Work out the finished part from the listing and answer in its coordinate system (mm). A direction names the side the tool comes from. Coordinates: 2 decimals unless noted, no trailing zeros. Write each loop counter-clockwise with the first axis right and the second up, starting at its lowest first coordinate (ties: lowest second). Pieces come first, ordered by that corner, then holes. Notation, with made-up numbers: (1, -6) - (41, -6) arc R5 cw to (41, 3) - close; hole circle Ø7 at (-37.75, -24). An arc over 180 degrees is marked (long way). Answer as a JSON object with one key per item and string values. Group by question number.
from build123d import *
from build123d.topology import SkipClean

# Parameters (mm, degrees)
EXTRUDE_1_DEPTH      = 4
EXTRUDE_1_DEPTH_BACK = 4
FILLET_4_R           = 1
EXTRUDE_2_DEPTH      = 5
FILLET_5_R           = 3
SKETCH_5_R           = 0.2
CUT_EXTRUDE_1_DEPTH  = 54.051861419


with BuildPart() as part:
    # Эскиз1 → Бобышка-Вытянуть1 (new, two sides: drawn at the far end of the back side and taken through both)
    with BuildSketch(Plane(origin=(22.5, -18, -41), x_dir=(0, -1, 0), z_dir=(1, 0, 0)).offset(-EXTRUDE_1_DEPTH_BACK)):
        with BuildLine():
            Line((-51, -2.5), (-51, 0.5))
            Line((-51, 0.5), (-61, 0.5))
            Line((-61, 0.5), (-61, -39.5))
            Line((-61, -39.5), (-51, -39.5))
            Line((-51, -39.5), (-51, -36.5))
            Line((-51, -36.5), (-58, -36.5))
            Line((-58, -36.5), (-58, -33.885132318))
            ThreePointArc((-58, -33.885132318), (-54.5, -35), (-51, -33.885132318))
            Line((-51, -33.885132318), (-51, -30.885132318))
            ThreePointArc((-51, -30.885132318), (-54.5, -32.948640645), (-58, -30.885132318))
            Line((-58, -30.885132318), (-58, -8.114867682))
            ThreePointArc((-58, -8.114867682), (-54.5, -6.051359355), (-51, -8.114867682))
            Line((-51, -8.114867682), (-51, -5.114867682))
            ThreePointArc((-51, -5.114867682), (-54.5, -4), (-58, -5.114867682))
            Line((-58, -5.114867682), (-58, -2.5))
            Line((-58, -2.5), (-51, -2.5))
        make_face()
    extrude(amount=EXTRUDE_1_DEPTH + EXTRUDE_1_DEPTH_BACK)

    # Скругление4
    # the kernel refuses this fillet: 1 mm, written as the material it adds along each edge
    with BuildSketch(Plane(origin=(26.5, 40, -38.5), x_dir=(0, 0, 1), z_dir=(-1, 0, 0)), Plane(origin=(18.5, 40, -4.5), x_dir=(0, 0, -1), z_dir=(1, 0, 0))) as fillet_4_piece_1:
        with BuildLine():
            CenterArc((FILLET_4_R, -FILLET_4_R), FILLET_4_R, 90, 90)
            Line((0, -FILLET_4_R), (0, 0))
            Line((0, 0), (FILLET_4_R, 0))
        make_face()
    extrude(amount=8)
    with BuildSketch(Plane(origin=(26.5, 40, -35.885132318), x_dir=(0, 0, -1), z_dir=(-1, 0, 0))) as fillet_4_piece_2:
        with BuildLine():
            CenterArc((1.65681317, 1), FILLET_4_R, 159.234649254, 110.765350746)
            ThreePointArc((0.721772915, 1.354541568), (0.404005567, 0.654294593), (0, 0))
            Line((0, 0), (1.65681317, 0))
        make_face()
    extrude(amount=8)
    with BuildSketch(Plane(origin=(18.5, 40, -32.885132318), x_dir=(0, -0.5188652741265531, -0.8548560272382577), z_dir=(1, 0, 0))) as fillet_4_piece_3:
        with BuildLine():
            CenterArc((0.281062042, -0.999193595), FILLET_4_R, 87.698857305, 33.557309762)
            Line((-0.237803232, -0.144337567), (0, 0))
            ThreePointArc((0, 0), (0.160606881, 0.003225622), (0.321213762, 0))
        make_face()
    extrude(amount=8)
    with BuildSketch(Plane(origin=(18.5, 40, -10.114867682), x_dir=(0, 0, -1), z_dir=(1, 0, 0))) as fillet_4_piece_4:
        with BuildLine():
            CenterArc((0.278179278, -1), FILLET_4_R, 90, 33.557309762)
            ThreePointArc((-0.27459152, -0.166666667), (-0.138969423, -0.080575891), (0, 0))
            Line((0, 0), (0.278179278, 0))
        make_face()
    extrude(amount=8)
    with BuildSketch(Plane(origin=(18.5, 40, -7.114867682), x_dir=(0, -0.8825285241752726, 0.4702588691529541), z_dir=(1, 0, 0))) as fillet_4_piece_5:
        with BuildLine():
            CenterArc((1.661659612, -0.991926012), FILLET_4_R, 97.285750856, 110.765350746)
            Line((0.779131087, -1.462184881), (0, 0))
            ThreePointArc((0, 0), (0.767420843, -0.048858602), (1.534841686, 0))
        make_face()
    extrude(amount=8)
    # the kernel refuses this fillet: 1 mm, written as the material it takes off along each edge
    with BuildSketch(Plane(origin=(17.002810413, 33, -35.885132318), x_dir=(0, 0, 1), z_dir=(1, 0, 0))) as fillet_4_2_piece_1:
        with BuildLine():
            CenterArc((0.547160138, -1), FILLET_4_R, 90, 60.33576985)
            ThreePointArc((-0.321780523, -0.505083716), (-0.167142324, -0.248558772), (0, 0))
            Line((0, 0), (0.547160138, 0))
        make_face()
    extrude(amount=10.994379174, mode=Mode.SUBTRACT)
    with BuildSketch(Plane(origin=(12.515911635, 33, -32.885132318), x_dir=(0, 0.7006292692220382, -0.7135254915624197), z_dir=(1, 0, 0))) as fillet_4_2_piece_2:
        with BuildLine():
            CenterArc((2.408549106, -0.963525492), FILLET_4_R, 105.522487814, 120)
            Line((1.707919837, -1.677050983), (0, 0))
            ThreePointArc((0, 0), (1.070466269, -0.145898034), (2.140932539, 0))
        make_face()
    extrude(amount=19.968176729, mode=Mode.SUBTRACT)
    with BuildSketch(Plane(origin=(12.515911635, 33, -10.114867682), x_dir=(0, 0, 1), z_dir=(1, 0, 0))) as fillet_4_2_piece_3:
        with BuildLine():
            CenterArc((2.393635346, -1), FILLET_4_R, 90, 120)
            ThreePointArc((1.527609942, -1.5), (0.866025404, -0.645898034), (0, 0))
            Line((0, 0), (2.393635346, 0))
        make_face()
    extrude(amount=19.968176729, mode=Mode.SUBTRACT)
    with BuildSketch(Plane(origin=(17.002810413, 33, -7.114867682), x_dir=(0, 0.8433863696195878, 0.5373075762911708), z_dir=(1, 0, 0))) as fillet_4_2_piece_4:
        with BuildLine():
            CenterArc((0.549393082, -0.998774978), FILLET_4_R, 87.163688846, 60.33576985)
            Line((-0.293993287, -0.461467402), (0, 0))
            ThreePointArc((0, 0), (0.299437917, 0.007413047), (0.598875835, 0))
        make_face()
    extrude(amount=10.994379174, mode=Mode.SUBTRACT)
    with BuildSketch(Plane(origin=(16, 33, -4.5), x_dir=(0, 0, 1), z_dir=(1, 0, 0)), Plane(origin=(16, 33, -1.5), x_dir=(0, 1, 0), z_dir=(1, 0, 0)), Plane(origin=(16, 43, -1.5), x_dir=(0, 0, -1), z_dir=(1, 0, 0)), Plane(origin=(16, 43, -41.5), x_dir=(0, -1, 0), z_dir=(1, 0, 0)), Plane(origin=(16, 33, -41.5), x_dir=(0, 0, 1), z_dir=(1, 0, 0)), Plane(origin=(29, 33, -38.5), x_dir=(0, 0, -1), z_dir=(-1, 0, 0))) as fillet_4_2_piece_5:
        with BuildLine():
            CenterArc((FILLET_4_R, -FILLET_4_R), FILLET_4_R, 90, 90)
            Line((0, -FILLET_4_R), (0, 0))
            Line((0, 0), (FILLET_4_R, 0))
        make_face()
    extrude(amount=13, mode=Mode.SUBTRACT)

    # Эскиз3 → Бобышка-Вытянуть2 (add)
    with SkipClean():  # the faces are left unmerged after this step: merging them gives an invalid solid
        with BuildSketch(Plane(origin=(26.5, 0, 0), x_dir=(0, 0, -1), z_dir=(1, 0, 0))):
            with BuildLine():
                Line((10.393046959, 40), (10.393046959, 43))
                Line((10.393046959, 43), (2.5, 43))
                ThreePointArc((2.5, 43), (1.792893219, 42.707106781), (1.5, 42))
                Line((1.5, 42), (1.5, 34))
                ThreePointArc((1.5, 34), (1.792893219, 33.292893219), (2.5, 33))
                Line((2.5, 33), (3.5, 33))
                ThreePointArc((3.5, 33), (4.207106781, 33.292893219), (4.5, 34))
                Line((4.5, 34), (4.5, 39))
                ThreePointArc((4.5, 39), (4.78551671, 39.699652505), (5.479027256, 39.999780048))
                ThreePointArc((5.479027256, 39.999780048), (6.286931447, 39.559430985), (6.393094766, 38.645458432))
                ThreePointArc((6.393094766, 38.645458432), (6.0182377, 36.030539524), (6.793087158, 33.505083716))
                ThreePointArc((6.793087158, 33.505083716), (7.159492389, 33.135443384), (7.662027819, 33))
                Line((7.662027819, 33), (7.721232336, 33))
                ThreePointArc((7.721232336, 33), (8.587257739, 33.5), (8.587257739, 34.5))
                ThreePointArc((8.587257739, 34.5), (8.157384295, 37.414854216), (9.840276161, 39.833333333))
                ThreePointArc((9.840276161, 39.833333333), (10.104371825, 39.957427108), (10.393046959, 40))
            make_face()
            with BuildLine():
                Line((32.606953041, 40), (32.606953041, 43))
                Line((32.606953041, 43), (40.5, 43))
                ThreePointArc((40.5, 43), (41.207106781, 42.707106781), (41.5, 42))
                Line((41.5, 42), (41.5, 34))
                ThreePointArc((41.5, 34), (41.207106781, 33.292893219), (40.5, 33))
                Line((40.5, 33), (39.5, 33))
                ThreePointArc((39.5, 33), (38.792893219, 33.292893219), (38.5, 34))
                Line((38.5, 34), (38.5, 39))
                ThreePointArc((38.5, 39), (38.21448329, 39.699652505), (37.520972744, 39.999780048))
                ThreePointArc((37.520972744, 39.999780048), (36.713068553, 39.559430985), (36.606905234, 38.645458432))
                ThreePointArc((36.606905234, 38.645458432), (36.9817623, 36.030539524), (36.206912842, 33.505083716))
                ThreePointArc((36.206912842, 33.505083716), (35.840507611, 33.135443384), (35.337972181, 33))
                Line((35.337972181, 33), (35.278767664, 33))
                ThreePointArc((35.278767664, 33), (34.412742261, 33.5), (34.412742261, 34.5))
                ThreePointArc((34.412742261, 34.5), (34.842615705, 37.414854216), (33.159723839, 39.833333333))
                ThreePointArc((33.159723839, 39.833333333), (32.895628175, 39.957427108), (32.606953041, 40))
            make_face()
        extrude_2 = extrude(amount=EXTRUDE_2_DEPTH)

    # Зеркальное отражение1: Бобышка-Вытянуть2 across plane
    with SkipClean():  # the faces are left unmerged after this step: merging them gives an invalid solid
        add(extrude_2.mirror(Plane(origin=(22.5, 0, 0), x_dir=(0, 0, 1), z_dir=(1, 0, 0))))

    # Скругление5
    # the kernel refuses this fillet: 3 mm, written as the material it adds along each edge
    with BuildSketch(Plane(origin=(26.5, 40, -32.606953041), x_dir=(0, 0, 1), z_dir=(0, 1, 0)), Plane(origin=(26.5, 40, -10.393046959), x_dir=(1, 0, 0), z_dir=(0, 1, 0))) as fillet_5_piece_1:
        with BuildLine():
            CenterArc((FILLET_5_R, FILLET_5_R), FILLET_5_R, 180, 90)
            Line((0, FILLET_5_R), (0, 0))
            Line((0, 0), (FILLET_5_R, 0))
        make_face()
    extrude(amount=3)
    with BuildSketch(Plane(origin=(18.5, 40, -32.606953041), x_dir=(0, 0, 1), z_dir=(0, 1, 0)), Plane(origin=(18.5, 40, -10.393046959), x_dir=(-1, 0, 0), z_dir=(0, 1, 0))) as fillet_5_piece_2:
        with BuildLine():
            CenterArc((FILLET_5_R, -FILLET_5_R), FILLET_5_R, 90, 90)
            Line((0, -FILLET_5_R), (0, 0))
            Line((0, 0), (FILLET_5_R, 0))
        make_face()
    extrude(amount=3)

    # Эскиз5 → Вырез-Вытянуть1 (cut, through all)
    with BuildSketch(Plane(origin=(0, 43, 0), x_dir=(1, 0, 0), z_dir=(0, 1, 0))):
        with Locations(Location((22.5, 21.5, 0), (0, 0, 180))):
            Circle(SKETCH_5_R)
    extrude(amount=-CUT_EXTRUDE_1_DEPTH, mode=Mode.SUBTRACT)


solid = part.part
Q1. Flat-ended cylindrical pins translate along their axes: pin 1 Ø0.9 at (y, z) = (42, -21.5) entering from +X; pin 2 Ø3.5 at (y, z) = (42, -22.5) entering from -X. Find the tip coordinate at first contact, or state that the pin passes through.
Q2. For a pull along Z with two mould halves and no side action, classify faces 1 (the face through (22, 33, -3)), 2 (the face through (22, 38, -1.5)), 3 (the face through (22.37, 33.49, -8.58)) as +Z half, -Z half, draft (parallel to the pull), parting line (faces both ways), or undercut.
Q3. Section B-B on z = -23 is taken. Determine the outline of the cut face in (x, y), plus the area to 3 significant figures.
Q4. A tool of negligible diameter and unlimited length cuts with its end or side. For faces 4 (the face through (17.645, 41.479, -31.705)), 5 (the face through (22, 33, -40)), 6 (the face through (22.374, 42.715, -1.801)), 7 (the face through (26.5, 42, -21)), 8 (the face through (23, 36, -38.5)), from which of +Z, -Z, +X, -X, +Y, -Y can it reach the whole face along a straight path? Write none if from no direction.
Q5. Consider L1, parallel to Z at x = 25.5, y = 36.25; L2, parallel to X at y = 42.2, z = -21.5; L3, parallel to Z at x = 30.25, y = 34.5. Determine where each line is inside the solid, lowest interval first. Write a range as from..to.
Numbers:
{
 "1": {"pin 1": "stops at x = 26.5", "pin 2": "stops at x = 18.5"},
 "2": {"face 1": "draft", "face 2": "+Z half", "face 3": "undercut"},
 "3": {"outline": "(18.5, 40) - (26.5, 40) - (26.5, 43) - (18.5, 43) - close", "area": "24.0 mm²"},
 "4": {"face 4": "-X, +Y, -Y", "face 5": "+Z, -Z, +X, -X, -Y", "face 6": "+Z, +X, -X, +Y", "face 7": "+X, +Y, -Y", "face 8": "+X, -X, -Y"},
 "5": {"L1": "z = -41.5..-38.5, -36.99..-34.94, -8.06..-6.01, -4.5..-1.5", "L2": "x = 18.5..22.3, 22.7..26.5", "L3": "z = -41.5..-38.5, -36.66..-34.41, -8.59..-6.34, -4.5..-1.5"}
}
